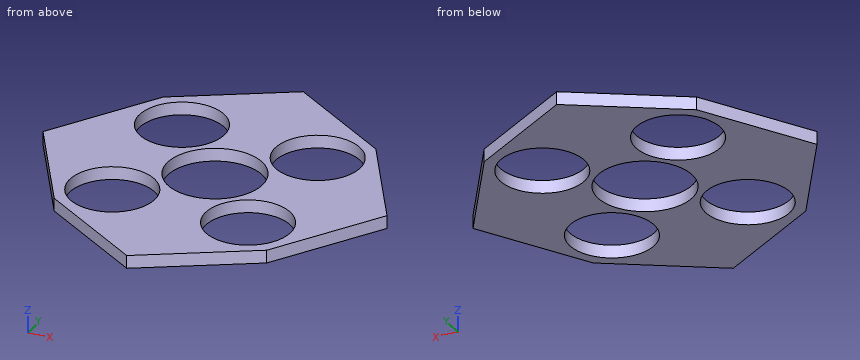
from build123d import *

# Parameters (mm, degrees)
F0_R     = 9.85
F0_R_2   = 11
F1_DEPTH = 3


with BuildPart() as f1:
    # F0 (on Top) → F1 (new body)
    with BuildSketch(Plane.XY):
        Polygon((24.715097, 24.715097), (0, 40), (-24.715097, 24.715097), (-40, 0), (-24.715097, -24.715097), (0, -40), (24.715097, -24.715097), (40, 0), align=None)
        with Locations((-15.78759, -15.78759)):
            Circle(F0_R, mode=Mode.SUBTRACT)
        with Locations((15.78759, -15.78759)):
            Circle(F0_R, mode=Mode.SUBTRACT)
        with Locations((-15.78759, 15.78759)):
            Circle(F0_R, mode=Mode.SUBTRACT)
        Circle(F0_R_2, mode=Mode.SUBTRACT)
        with Locations((15.78759, 15.78759)):
            Circle(F0_R, mode=Mode.SUBTRACT)
    extrude(amount=F1_DEPTH)


solid = f1.part
Model file for the job. Use its own axes, mm. Coordinates: 2 decimals unless noted, no trailing zeros. Order: outer loops, then holes, each group sorted by start corner. A loop starts at its lowest first (then second) coordinate and runs counter-clockwise, first axis right, second up. Notation, with made-up numbers: M 40,-32.75 L 83,-32.75 A22 ccw 83,-26.75 Z; hole C 73,61 d11. An arc over 180 degrees is marked long. Return JSON: item names as keys, results as strings.
1. Saw through at A-A (x = -17.5). Give the cut face in (y, z), and give its area (3 significant figures).
Ans:
{"outline": "M -29.18,0 L -25.49,0 L -25.49,3 L -29.18,3 Z; M -6.09,0 L 6.09,0 L 6.09,3 L -6.09,3 Z; M 25.49,0 L 29.18,0 L 29.18,3 L 25.49,3 Z", "area": "58.7 mm^2"}
2. Saw through at D-D (x = 2.5). Give the cut face in (y, z), and give its area (3 significant figures).
Ans:
{"outline": "M -38.45,0 L -10.71,0 L -10.71,3 L -38.45,3 Z; M 10.71,0 L 38.45,0 L 38.45,3 L 10.71,3 Z", "area": "166 mm^2"}
3. Saw through at B-B (y = -12.5). Give the cut face in (x, z).
Ans:
{"outline": "M -32.27,0 L -25.07,0 L -25.07,3 L -32.27,3 Z; M -6.5,0 L 6.5,0 L 6.5,3 L -6.5,3 Z; M 25.07,0 L 32.27,0 L 32.27,3 L 25.07,3 Z"}
4. Drill centre lines: probe 1 along X at (y, z) = (9, 2); probe 2 along Y at (x, z) = (14, 2.3); probe 3 along X at (y, z) = (-8, 1.6). Where is each one in solid material? Low to high.
Ans:
{"probe 1": "-34.43 to -22.93, -8.65 to -6.32, 6.32 to 8.65, 22.93 to 34.43", "probe 2": "-31.34 to -25.47, -6.1 to 6.1, 25.47 to 31.34", "probe 3": "-35.05 to -21.82, -9.76 to -7.55, 7.55 to 9.76, 21.82 to 35.05"}
5. Saw through at C-C (y = 9). Give the cut face in (x, z).
Ans:
{"outline": "M -34.43,0 L -22.93,0 L -22.93,3 L -34.43,3 Z; M -8.65,0 L -6.32,0 L -6.32,3 L -8.65,3 Z; M 6.32,0 L 8.65,0 L 8.65,3 L 6.32,3 Z; M 22.93,0 L 34.43,0 L 34.43,3 L 22.93,3 Z"}
6. Flat gauge pins, fed straight in: pin 1 (22.5 mm diameter, centred on x = -15.79, y = 15.79, fed in from +Z); pin 2 (1.5 mm diameter, centred on x = -28, z = 1.5, fed in from -Y). Where does each tip first touch, or does it go through?
Ans:
{"pin 1": "z = 3", "pin 2": "y = -20.62"}
